```python
from build123d import *

# Parameters (mm, degrees)
BOSS_EXTRUDE1_DEPTH      = 8.49
BOSS_EXTRUDE1_DEPTH_BACK = 2


with BuildPart() as part:
    # Sketch5 → Boss-Extrude1 (new, two sides: drawn at the far end of the back side and taken through both)
    with BuildSketch(Plane.XY.offset(-BOSS_EXTRUDE1_DEPTH_BACK)):
        with BuildLine():
            add(Edge.make_bspline(
                [(-6.214416506, 150), (-0.083680578, 146.836659722), (12.227049193, 121.171627413), (22.115504043, 97.266361341), (23.975, 92.038961998)],
                knots=[0.59541155, 0.59541155, 0.59541155, 0.59541155, 0.789536521, 0.848897281, 0.848897281, 0.848897281, 0.848897281], degree=3))
            Line((-6.214416506, 150), (-9.181360733, 150))
            add(Edge.make_bspline(
                [(-23.975, 97.550523877), (-22.525140626, 102.797342224), (-14.830547849, 121.396895041), (-13.344437158, 147.084687463), (-9.181360733, 150)],
                knots=[0.316420869, 0.316420869, 0.316420869, 0.316420869, 0.391637385, 0.56041045, 0.56041045, 0.56041045, 0.56041045], degree=3))
            Line((-23.975, 97.550523877), (-23.975, -31.128230966))
            add(Edge.make_bspline(
                [(-23.975, -31.128230966), (-21.293057089, -31.780629914), (-13.925723024, -33.572778799), (-8.294753832, -44.012214815), (-7.791781952, -51.627914113), (-7.595916378, -54.593593445)],
                knots=[0, 0, 0, 0, 0.258985483, 0.711436685, 1, 1, 1, 1], degree=3))
            Line((-7.595916378, -54.593593445), (-7.595916378, -150))
            Line((-7.595916378, -150), (7.595916378, -150))
            Line((7.595916378, -150), (7.595916378, -54.593593445))
            add(Edge.make_bspline(
                [(23.975, -31.128230966), (21.293057089, -31.780629914), (13.925723024, -33.572778799), (8.294753832, -44.012214815), (7.791781952, -51.627914113), (7.595916378, -54.593593445)],
                knots=[0, 0, 0, 0, 0.258985483, 0.711436685, 1, 1, 1, 1], degree=3))
            Line((23.975, -31.128230966), (23.975, 92.038961998))
        make_face()
    extrude(amount=BOSS_EXTRUDE1_DEPTH + BOSS_EXTRUDE1_DEPTH_BACK)


solid = part.part
```
Could you check a few things on this model? Use its own coordinates, in mm. A direction names the side the tool comes from. Round coordinates to 2 decimals unless told otherwise and drop trailing zeros. Write each loop counter-clockwise with the first axis right and the second up, starting at its lowest first coordinate (ties: lowest second). Pieces come first, ordered by that corner, then holes.
(1) If I drill on probe 1 along X at (y, z) = (-83, 7.75); probe 2 along Y at (x, z) = (0, 1); probe 3 along Y at (x, z) = (-10, 7.5), over which ranges is the centre line in solid material (lowest first)?
Findings below:
probe 1: x = -7.6 to 7.6
probe 2: y = -150 to 143.27
probe 3: y = -41.91 to 149.19
(2) For pin 1 (6 mm diameter, centred on x = 4, z = 1.5, fed in from +Y); pin 2 (3 mm diameter, centred on y = -79, z = 1, fed in from +X); pin 3 (5 mm diameter, centred on y = -95, z = 2.5, fed in from -X); pin 4 (4 mm diameter, centred on x = -10.5, z = 5, fed in from +Y), each with a flat end and sliding along its axis, tell me the tip position at first contact or that it passes through.
Findings below:
pin 1: stops at y = 141.74
pin 2: stops at x = 7.6
pin 3: stops at x = -7.6
pin 4: stops at y = 150
(3) Suppose I cut it at A-A on y = -99.5. Write out the boundary of the cut face in (x, z).
Findings below:
outline: (-7.6, -2) - (7.6, -2) - (7.6, 8.49) - (-7.6, 8.49) - close
(4) Which directions (+Z, -Z, +X, -X, +Y, -Y) give clear straight access to the entire face, cutting with the end or side of a thin tool? Please do faces 1 (the face through (-7.596, -102, 3)), 2 (the face through (7.596, -103, 3)), 3 (the face through (23.975, 30, 3)).
Findings below:
face 1: +Z, -Z, -X, -Y
face 2: +Z, -Z, +X, -Y
face 3: +Z, -Z, +X, +Y, -Y
